Can you work these out from the model? Positions are in its coordinate system, mm. Face numbers are marked on the shaded views. A direction names the side the tool comes from. Give positions to 0.01 mm unless a question says otherwise; leave off trailing zeros. Order: outer loops, then holes, each group sorted by start corner. A loop starts at its lowest first (then second) coordinate and runs counter-clockwise, first axis right, second up. Notation, with made-up numbers: (45.5, 21) - (81.5, 21) arc R20 ccw to (81.5, 27) - close; hole circle Ø2 at (77, -20). An arc over 180 degrees is marked (long way). Answer as CSV lines item,"result".
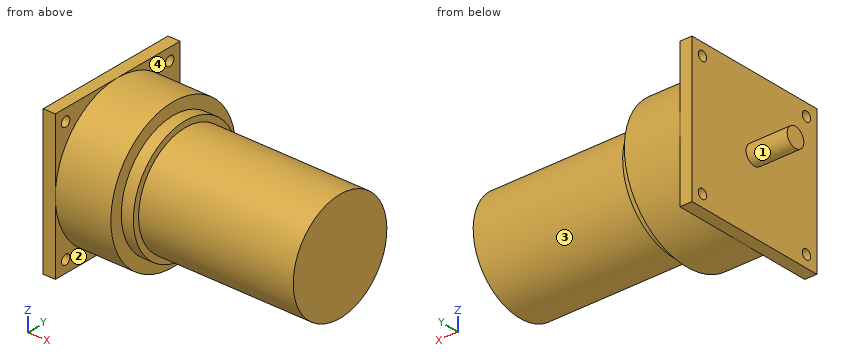
```python
from build123d import *

# Parameters (mm, degrees)
SKETCH2_W           = 60
SKETCH2_H           = 60
SKETCH2_R           = 2
BOSS_EXTRUDE1_DEPTH = 5


with BuildPart() as part:
    # Sketch1 → Revolve1 (revolve)
    with BuildSketch(Plane(origin=(0, 0, 0), x_dir=(1, 0, 0), z_dir=(0, 1, 0)), mode=Mode.PRIVATE) as revolve1_sk:
        Polygon((0, 0), (0, 4), (19, 4), (19, 12), (22, 12), (22, 30), (45, 30), (45, 25), (50, 25), (50, 22.5), (114, 22.5), (114, 0), align=None)
    revolve(revolve1_sk.sketch.rotate(Axis((0, 0, 0), (1, 0, 0)), 180), axis=Axis((0, 0, 0), (1, 0, 0)))

    # Sketch2 → Boss-Extrude1 (add)
    with BuildSketch(Plane.ZY.offset(-22)):
        Rectangle(SKETCH2_W, SKETCH2_H)
        with Locations((-25, 25)):
            Circle(SKETCH2_R, mode=Mode.SUBTRACT)
        with Locations((25, 25)):
            Circle(SKETCH2_R, mode=Mode.SUBTRACT)
        with Locations((25, -25)):
            Circle(SKETCH2_R, mode=Mode.SUBTRACT)
        with Locations((-25, -25)):
            Circle(SKETCH2_R, mode=Mode.SUBTRACT)
    extrude(amount=BOSS_EXTRUDE1_DEPTH)


solid = part.part
```
1) I want a section at A-A on z = -18. Write out the boundary of the cut face in (x, y).
Answer block:
outline,"(17, -30) - (22, -30) - (22, -24) - (45, -24) - (45, -17.35) - (50, -17.35) - (50, -13.5) - (114, -13.5) - (114, 13.5) - (50, 13.5) - (50, 17.35) - (45, 17.35) - (45, 24) - (22, 24) - (22, 30) - (17, 30) - close"
2) I'm going to push flat-ended pins straight in: P1, Ø1.5, axis at y = 22.5, z = -5.5, coming from the -X side; P2, Ø6, axis at x = 93, z = 15.5, coming from the -Y side; P3, Ø3.5, axis at y = 25, z = -25, coming from the -X side; P4, Ø6, axis at x = 69, z = 14.5, coming from the -Y side. Where does each tip first touch, or does it pass through?
Answer block:
P1,"x = 17"
P2,"y = -18.71"
P3,"through"
P4,"y = -19.34"
3) I want a section at C-C on x = 89. Write out the boundary of the cut face in (y, z).
Answer block:
outline,"circle Ø45 at (0, 0)"
4) Which directions (+Z, -Z, +X, -X, +Y, -Y) give clear straight access to the entire face, cutting with the end or side of a thin tool? Please do the marked faces 1, 2, 3 and 4.
Answer block:
face 1,"-X"
face 2,"-Z, +X, -Y"
face 3,"+X"
face 4,"+Z, +X, +Y"
5) I need wall thicknesses on line 1 along Y through (x, z) = (20.65, -25); line 2 along X through (y, z) = (26, -1.5); line 3 along X through (y, z) = (-7, 3). Which ranges of each line are inside material? Lowest first, please. Write a range as [from, to].
Answer block:
line 1,"[-30, -27], [-23, 23], [27, 30]"
line 2,"[17, 45]"
line 3,"[17, 114]"
6) I want a section at D-D on y = -2. Write out the boundary of the cut face in (x, z).
Answer block:
outline,"(0, -3.46) - (17, -3.46) - (17, -30) - (22, -30) - (22, -29.93) - (45, -29.93) - (45, -24.92) - (50, -24.92) - (50, -22.41) - (114, -22.41) - (114, 22.41) - (50, 22.41) - (50, 24.92) - (45, 24.92) - (45, 29.93) - (22, 29.93) - (22, 30) - (17, 30) - (17, 3.46) - (0, 3.46) - close"
7) I want a section at B-B on y = -18.5. Write out the boundary of the cut face in (x, z).
Answer block:
outline,"(17, -30) - (22, -30) - (22, -23.62) - (45, -23.62) - (45, -16.82) - (50, -16.82) - (50, -12.81) - (114, -12.81) - (114, 12.81) - (50, 12.81) - (50, 16.82) - (45, 16.82) - (45, 23.62) - (22, 23.62) - (22, 30) - (17, 30) - close"
